The listing builds one solid part. Answer for the finished solid, in the listing's coordinates (mm). Give positions to 0.01 mm unless a question says otherwise; leave off trailing zeros. Write each question's results on one line, items separated by ' | '. Start each with the question number.
Q1. Find the intervals of material crossed by probe 1 along Z at (x, y) = (1, 308.5); probe 2 along Z at (x, y) = (0.5, 104); probe 3 along Z at (x, y) = (2, 144), in increasing order.
Q2. Flat-ended cylindrical pins translate along their axes: pin 1 Ø4 at (y, z) = (255.5, -247) entering from -X; pin 2 Ø3 at (x, y) = (3, 47.5) entering from -Z; pin 3 Ø3 at (x, z) = (2.5, -258) entering from +Y; pin 4 Ø4 at (y, z) = (256.52, 147.96) entering from -X. Find the tip coordinate at first contact, or state that the pin passes through.
Q3. Section A-A (x = 4) is taken. State how many separate pieces and enclosed holes the cut face has, plus the area to 3 significant figures.
```python
from build123d import *
from OCP.BRepFilletAPI import BRepFilletAPI_MakeChamfer

# Parameters (mm, degrees)
BOSS_EXTRUDE1_DEPTH                            = 6.35
SKETCH2_W                                      = 25.4
SKETCH2_H                                      = 304.8
CUT_EXTRUDE1_DEPTH                             = 672.86027017
FILLET1_R                                      = 6.35
CHAMFER3_SIZE                                  = 3.666174209
CHAMFER3_SIZE_2                                = 6.35
CSK_FOR_4_FLAT_HEAD_MACHINE_SCREW1_D           = 3.2639
CSK_FOR_4_FLAT_HEAD_MACHINE_SCREW1_CSINK_D     = 5.715
CSK_FOR_4_FLAT_HEAD_MACHINE_SCREW1_CSINK_ANGLE = 82
CUT_EXTRUDE2_REACH                             = 669.791
CSK_FOR_4_FLAT_HEAD_MACHINE_SCREW2_D           = 3.2639
CSK_FOR_4_FLAT_HEAD_MACHINE_SCREW2_CSINK_D     = 5.715
CSK_FOR_4_FLAT_HEAD_MACHINE_SCREW2_CSINK_ANGLE = 82


with BuildPart() as part:
    # Sketch1 → Boss-Extrude1 (new body)
    with BuildSketch(Plane(origin=(0, 0, 0), x_dir=(0, 0, -1), z_dir=(1, 0, 0))):
        Polygon((588.635764647, 323.826862244), (383.330008924, -31.773137756), (-160.664235353, -31.773137756), (-160.664235353, 323.826862244), align=None)
    extrude(amount=BOSS_EXTRUDE1_DEPTH)

    # Sketch2 → Cut-Extrude1 (cut, through all)
    with BuildSketch(Plane.ZY):
        with Locations((-258.435764647, 171.426862244)):
            Rectangle(SKETCH2_W, SKETCH2_H)
    extrude(amount=-CUT_EXTRUDE1_DEPTH, mode=Mode.SUBTRACT)

    # Fillet1
    fillet1_edges = [part.edges().sort_by_distance(p)[0] for p in [
        (3.175, 323.826862244, -588.635764647),
    ]]
    fillet(fillet1_edges, radius=FILLET1_R)

    # Chamfer3
    chamfer3_edges_1 = [part.edges().sort_by_distance(p)[0] for p in [
        (6.35, 323.826862244, -42.535764647),
    ]]
    chamfer3_side_1 = [part.faces().sort_by_distance(p)[0] for p in [
        (6.35, 323.753538759, -42.535764647),
    ]]
    chamfer3_edges_2 = [part.edges().sort_by_distance(p)[0] for p in [
        (6.35, 141.264362244, -483.233256128),
    ]]
    chamfer3_side_2 = [part.faces().sort_by_distance(p)[0] for p in [
        (6.276676516, 141.264362244, -483.233256128),
    ]]
    chamfer3_edges_3 = [part.edges().sort_by_distance(p)[0] for p in [
        (6.35, 320.651862244, -583.136503333),
    ]]
    chamfer3_side_3 = [part.faces().sort_by_distance(p)[0] for p in [
        (6.276676516, 320.651862244, -583.136503333),
    ]]
    chamfer3_edges_4 = [part.edges().sort_by_distance(p)[0] for p in [
        (6.35, 323.826862244, -424.386503333),
    ]]
    chamfer3_side_4 = [part.faces().sort_by_distance(p)[0] for p in [
        (6.35, 323.753538759, -424.386503333),
    ]]
    chamfer3 = BRepFilletAPI_MakeChamfer(part.part.solid().wrapped)
    for e in chamfer3_edges_1:
        chamfer3.Add(CHAMFER3_SIZE - 0.0001, CHAMFER3_SIZE_2 - 0.0001, e.wrapped, chamfer3_side_1[0].wrapped)
    for e in chamfer3_edges_2:
        chamfer3.Add(CHAMFER3_SIZE_2 - 0.0001, CHAMFER3_SIZE - 0.0001, e.wrapped, chamfer3_side_2[0].wrapped)
    for e in chamfer3_edges_3:
        chamfer3.Add(CHAMFER3_SIZE_2 - 0.0001, CHAMFER3_SIZE - 0.0001, e.wrapped, chamfer3_side_3[0].wrapped)
    for e in chamfer3_edges_4:
        chamfer3.Add(CHAMFER3_SIZE - 0.0001, CHAMFER3_SIZE_2 - 0.0001, e.wrapped, chamfer3_side_4[0].wrapped)
    add(Compound.cast(chamfer3.Shape()), mode=Mode.REPLACE)  # a hair under: the kernel refuses the full size

    # CSK for #4 Flat Head Machine Screw1 (through all)
    with Locations(Plane(origin=(0, 256.516862244, 147.964235353), x_dir=(0, 0, -1), z_dir=(-1, 0, 0))):
        with Locations((0, 0), (317.5, -25.4), (469.9, -25.4), (0, 152.4), (63.5, 262.89), (317.5, 262.89)):
            CounterSinkHole(CSK_FOR_4_FLAT_HEAD_MACHINE_SCREW1_D / 2, CSK_FOR_4_FLAT_HEAD_MACHINE_SCREW1_CSINK_D / 2, counter_sink_angle=CSK_FOR_4_FLAT_HEAD_MACHINE_SCREW1_CSINK_ANGLE)

    # Sketch7 → Cut-Extrude2 (cut, up to next)
    with BuildSketch(Plane.ZY, mode=Mode.PRIVATE) as cut_extrude2_sk1:
        with BuildLine():
            Line((140.071185353, 89.635966927), (140.071185353, 83.285966927))
            ThreePointArc((140.071185353, 83.285966927), (138.439235353, 81.654016927), (136.807285353, 83.285966927))
            Line((136.807285353, 83.285966927), (136.807285353, 89.635966927))
            ThreePointArc((136.807285353, 89.635966927), (138.439235353, 91.267916927), (140.071185353, 89.635966927))
        make_face()
    cut_extrude2_tool1 = extrude(cut_extrude2_sk1.sketch, amount=-CUT_EXTRUDE2_REACH, mode=Mode.PRIVATE) & part.part
    # Sketch7 → Cut-Extrude2 (cut, up to next)
    with BuildSketch(Plane.ZY, mode=Mode.PRIVATE) as cut_extrude2_sk2:
        with BuildLine():
            Line((98.707285353, 83.285966927), (98.707285353, 89.635966927))
            ThreePointArc((98.707285353, 89.635966927), (100.339235353, 91.267916927), (101.971185353, 89.635966927))
            Line((101.971185353, 89.635966927), (101.971185353, 83.285966927))
            ThreePointArc((101.971185353, 83.285966927), (100.339235353, 81.654016927), (98.707285353, 83.285966927))
        make_face()
    cut_extrude2_tool2 = extrude(cut_extrude2_sk2.sketch, amount=-CUT_EXTRUDE2_REACH, mode=Mode.PRIVATE) & part.part
    # Sketch7 → Cut-Extrude2 (cut, up to next)
    with BuildSketch(Plane.ZY, mode=Mode.PRIVATE) as cut_extrude2_sk3:
        with BuildLine():
            Line((98.707285353, 45.185966927), (98.707285353, 51.535966927))
            ThreePointArc((98.707285353, 51.535966927), (100.339235353, 53.167916927), (101.971185353, 51.535966927))
            Line((101.971185353, 51.535966927), (101.971185353, 45.185966927))
            ThreePointArc((101.971185353, 45.185966927), (100.339235353, 43.554016927), (98.707285353, 45.185966927))
        make_face()
    cut_extrude2_tool3 = extrude(cut_extrude2_sk3.sketch, amount=-CUT_EXTRUDE2_REACH, mode=Mode.PRIVATE) & part.part
    # Sketch7 → Cut-Extrude2 (cut, up to next)
    with BuildSketch(Plane.ZY, mode=Mode.PRIVATE) as cut_extrude2_sk4:
        with BuildLine():
            Line((136.807285353, 45.185966927), (136.807285353, 51.535966927))
            ThreePointArc((136.807285353, 51.535966927), (138.439235353, 53.167916927), (140.071185353, 51.535966927))
            Line((140.071185353, 51.535966927), (140.071185353, 45.185966927))
            ThreePointArc((140.071185353, 45.185966927), (138.439235353, 43.554016927), (136.807285353, 45.185966927))
        make_face()
    cut_extrude2_tool4 = extrude(cut_extrude2_sk4.sketch, amount=-CUT_EXTRUDE2_REACH, mode=Mode.PRIVATE) & part.part
    add(cut_extrude2_tool1.solids().sort_by_distance((0, 86.460967, 138.439235))[0], mode=Mode.SUBTRACT)
    add(cut_extrude2_tool2.solids().sort_by_distance((0, 86.460967, 100.339235))[0], mode=Mode.SUBTRACT)
    add(cut_extrude2_tool3.solids().sort_by_distance((0, 48.360967, 100.339235))[0], mode=Mode.SUBTRACT)
    add(cut_extrude2_tool4.solids().sort_by_distance((0, 48.360967, 138.439235))[0], mode=Mode.SUBTRACT)

    # CSK for #4 Flat Head Machine Screw2 (through all)
    with Locations(Plane.ZY):
        with Locations((132.089235353, 307.460688034), (144.789235353, 307.460688034)):
            CounterSinkHole(CSK_FOR_4_FLAT_HEAD_MACHINE_SCREW2_D / 2, CSK_FOR_4_FLAT_HEAD_MACHINE_SCREW2_CSINK_D / 2, counter_sink_angle=CSK_FOR_4_FLAT_HEAD_MACHINE_SCREW2_CSINK_ANGLE)


solid = part.part
```
Answers below:
1) probe 1: z = -579.12 to -271.14, -245.74 to 130.39, 133.78 to 143.09, 146.48 to 160.66 | probe 2: z = -461.39 to -271.14, -245.74 to 145.54, 150.38 to 160.66 | probe 3: z = -483.48 to -271.14, -245.74 to 160.66
2) pin 1: stops at x = 0 | pin 2: stops at z = -428.42 | pin 3: stops at y = 19.03 | pin 4: stops at x = 0.98
3) separate pieces: 1 | enclosed holes: 12 | area: 219,000 mm2
